Input: part model. Units: mm. Frame: model coordinates. Round coordinates to 2 decimals unless told otherwise and drop trailing zeros. Write each loop counter-clockwise with the first axis right and the second up, starting at its lowest first coordinate (ties: lowest second). Pieces come first, ordered by that corner, then holes. Notation, with made-up numbers: (47, -15) -> (76, -15) arc R29 ccw to (76, 7) -> close; hole circle Ø3 at (-20, 68). An arc over 180 degrees is marked (long way). Use CSV: the item, a comma, the result in double quotes.
```python
from build123d import *

# Parameters (mm, degrees)
SKETCH_1_W          = 50
SKETCH_1_H          = 30
EXTRUDE_1_DEPTH     = 3
SKETCH_2_R          = 2.6
SKETCH_2_R_2        = 1.6
SKETCH_2_R_3        = 5.25
CUT_EXTRUDE_1_DEPTH = 5


with BuildPart() as part:
    # 草图1 → 凸台-拉伸1 (new body)
    with BuildSketch(Plane.XY):
        with Locations((25, 15)):
            Rectangle(SKETCH_1_W, SKETCH_1_H)
    extrude(amount=EXTRUDE_1_DEPTH)

    # 草图2 → 切除-拉伸1 (cut)
    with BuildSketch(Plane.XY.offset(3)):
        with Locations((8, 15)):
            Circle(SKETCH_2_R)
        with Locations((42, 15)):
            Circle(SKETCH_2_R)
        with Locations((30.656854249, 20.656854249)):
            Circle(SKETCH_2_R_2)
        with Locations((30.656854249, 9.343145751)):
            Circle(SKETCH_2_R_2)
        with Locations((19.343145751, 9.343145751)):
            Circle(SKETCH_2_R_2)
        with Locations((19.343145751, 20.656854249)):
            Circle(SKETCH_2_R_2)
        with Locations((25, 15)):
            Circle(SKETCH_2_R_3)
        with Locations((45, 3.734603705)):
            Circle(SKETCH_2_R_2)
        with Locations(Location((45, 26.265396295, 0), (0, 0, 180))):
            Circle(SKETCH_2_R_2)
        with Locations((5, 26.265396295)):
            Circle(SKETCH_2_R_2)
        with Locations(Location((5, 3.734603705, 0), (0, 0, 180))):
            Circle(SKETCH_2_R_2)
    extrude(amount=-CUT_EXTRUDE_1_DEPTH, mode=Mode.SUBTRACT)


solid = part.part
```
Item 1: Section query A-A on x = 25. Return the cut outline in (y, z).
Worked answers:
outline,"(0, 0) -> (9.75, 0) -> (9.75, 3) -> (0, 3) -> close; (20.25, 0) -> (30, 0) -> (30, 3) -> (20.25, 3) -> close"
Item 2: Line query: line 1 (Y direction, x = 45, z = 1.3); line 2 (X direction, y = 3.75, z = 2.1); line 3 (Y direction, x = 25, z = 1.8). Output: solid intervals per line, ascending.
Worked answers:
line 1,"y = 0 to 2.13, 5.33 to 24.67, 27.87 to 30"
line 2,"x = 0 to 3.4, 6.6 to 43.4, 46.6 to 50"
line 3,"y = 0 to 9.75, 20.25 to 30"
Item 3: First-contact query: pin 1 Ø6.5 at (x, y) = (25, 15) entering from +Z. Flat tip, straight axial feed; report the tip coordinate or a pass-through.
Worked answers:
pin 1,"passes through"
Item 4: Section query D-D on x = 31. Return the cut outline in (y, z).
Worked answers:
outline,"(0, 0) -> (7.78, 0) -> (7.78, 3) -> (0, 3) -> close; (10.91, 0) -> (19.09, 0) -> (19.09, 3) -> (10.91, 3) -> close; (22.22, 0) -> (30, 0) -> (30, 3) -> (22.22, 3) -> close"
Item 5: Section query C-C on z = 2. Give the number of separate pieces and of enclosed holes in the cut face, plus the area to 3 significant figures.
Worked answers:
separate pieces,"1"
enclosed holes,"11"
area,"1,310 mm²"
Item 6: Section query B-B on y = 15. Return the cut outline in (x, z).
Worked answers:
outline,"(0, 0) -> (5.4, 0) -> (5.4, 3) -> (0, 3) -> close; (10.6, 0) -> (19.75, 0) -> (19.75, 3) -> (10.6, 3) -> close; (30.25, 0) -> (39.4, 0) -> (39.4, 3) -> (30.25, 3) -> close; (44.6, 0) -> (50, 0) -> (50, 3) -> (44.6, 3) -> close"
Item 7: Pull-direction query (X, two-part tool) for faces 1 (the face through (5.347, 5.297, 1.521)), 2 (the face through (19, 15, 3)), 3 (the face through (50, 15, 1)); classes: +X half, -X half, draft (parallel to the pull), parting line (faces both ways), or undercut.
Worked answers:
face 1,"undercut"
face 2,"draft"
face 3,"+X half"
